Verification items for the finished model (mm, model axes). A direction names the side the tool comes from. Coordinates: 2 decimals unless noted, no trailing zeros. Order: outer loops, then holes, each group sorted by start corner. A loop starts at its lowest first (then second) coordinate and runs counter-clockwise, first axis right, second up. Notation, with made-up numbers: M 32.25,51 L 79.25,51 A15 cw 79.25,59 Z; hole C 24,2.5 d5. An arc over 180 degrees is marked long. Use one line per item in the form item = value. Start each with the question number.
```python
from build123d import *

# Parameters (mm, degrees)
CROQUIS1_W              = 50.8
CROQUIS1_H              = 25.5016
SALIENTE_EXTRUIR1_DEPTH = 3.175
CROQUIS2_W              = 25.5016
CROQUIS2_H              = 46.3804
SALIENTE_EXTRUIR2_DEPTH = 18.3388
CORTAR_EXTRUIR2_DEPTH   = 13.26
SALIENTE_EXTRUIR3_DEPTH = 1.27
CROQUIS6_W              = 25.5016
CROQUIS6_H              = 46.3804
SALIENTE_EXTRUIR4_DEPTH = 2.54
CROQUIS7_W              = 25.5016
CROQUIS7_H              = 3.175
SALIENTE_EXTRUIR5_DEPTH = 50.8
CROQUIS8_W              = 72.9488
CROQUIS8_H              = 46.3804
SALIENTE_EXTRUIR6_DEPTH = 3.175


with BuildPart() as part:
    # Croquis1 → Saliente-Extruir1 (new body)
    with BuildSketch(Plane(origin=(0, 23.1902, 0), x_dir=(1, 0, 0), z_dir=(0, 1, 0))):
        with Locations((76.2, 0)):
            Rectangle(CROQUIS1_W, CROQUIS1_H)
    extrude(amount=-SALIENTE_EXTRUIR1_DEPTH)

    # Croquis2 → Saliente-Extruir2 (add)
    with BuildSketch(Plane(origin=(101.6, 0, 0), x_dir=(0, 0, -1), z_dir=(1, 0, 0))):
        Rectangle(CROQUIS2_W, CROQUIS2_H)
    extrude(amount=SALIENTE_EXTRUIR2_DEPTH)

    # Croquis4 → Cortar-Extruir2 (cut)
    with BuildSketch(Plane(origin=(0, 7.26, 0), x_dir=(1, 0, 0), z_dir=(0, 1, 0))):
        Polygon((104.14, -5.08), (104.14, -12.7508), (116.94, -12.7508), (116.94, -9.1694), (119.9388, -6.6294), (119.9388, 6.6294), (116.94, 9.1694), (116.94, 12.7508), (104.14, 12.7508), (104.14, 5.08), (101.6, 2.54), (101.6, -2.54), align=None)
    extrude(amount=-CORTAR_EXTRUIR2_DEPTH, mode=Mode.SUBTRACT)

    # Croquis5 → Saliente-Extruir3 (add)
    with BuildSketch(Plane(origin=(119.9388, 0, 0), x_dir=(0, 0, -1), z_dir=(1, 0, 0))):
        Polygon((-12.7508, -23.1902), (-12.7508, -19.9644), (12.7, -19.9644), (12.7, 19.9644), (-12.7508, 19.9644), (-12.7508, 23.1902), (12.7508, 23.1902), (12.7508, -23.1902), align=None)
    extrude(amount=SALIENTE_EXTRUIR3_DEPTH)

    # Croquis6 → Saliente-Extruir4 (add)
    with BuildSketch(Plane(origin=(121.2088, 0, 0), x_dir=(0, 0, -1), z_dir=(1, 0, 0))):
        Rectangle(CROQUIS6_W, CROQUIS6_H)
        Polygon((6.651353306, 1.27), (6.651353306, 13.8938), (-6.607446694, 13.8938), (-6.607446694, -13.8938), (6.651353306, -13.8938), align=None, mode=Mode.SUBTRACT)
    extrude(amount=SALIENTE_EXTRUIR4_DEPTH)

    # Croquis7 → Saliente-Extruir5 (add)
    with BuildSketch(Plane.ZY.offset(-101.6)):
        with Locations((0, -21.6027)):
            Rectangle(CROQUIS7_W, CROQUIS7_H)
    extrude(amount=SALIENTE_EXTRUIR5_DEPTH)

    # Croquis8 → Saliente-Extruir6 (add)
    with BuildSketch(Plane(origin=(0, 0, -12.7508), x_dir=(-1, 0, 0), z_dir=(0, 0, -1))):
        with Locations((-87.2744, 0)):
            Rectangle(CROQUIS8_W, CROQUIS8_H)
    extrude(amount=SALIENTE_EXTRUIR6_DEPTH)


solid = part.part
```
1. Cross-section at D-D on x = 62. Enter the section's corners in (y, z), and give its area (3 significant figures).
2. Cross-section at B-B on z = -0.5. Enter the section's corners in (x, y).
3. Cross-section at A-A on y = 2.5. Enter the section's corners in (x, z).
4. Material ranges on line 1 along X through (y, z) = (3, -12); line 2 along Y through (x, z) = (67.5, 6.5); line 3 along X through (y, z) = (19.5, 10.5), recorded low to high.
5. Cross-section at C-C on z = -10. Enter the section's corners in (x, y).
6. Release check for a two-part mould opening along Z. For faces 1 (the flat face through (122, 13.894, 0)), 2 (the flat face through (77, -20.015, 0)), 3 (the flat face through (103.7, -0.1, 12.751)) record: pulls with the +Z half, pulls with the -Z half, needs draft (parallel to the pull), parting line crosses it, or undercut.
7. Tool access check on faces 4 (the flat face through (76, 20.015, 0)), 5 (the flat face through (122, 0, 6.607)), 6 (the flat face through (88, -23.19, -1)), 7 (the flat face through (104.14, 1, 9)), 8 (the flat face through (118.418, 0.723, 7.917)). Record the directions out of +Z, -Z, +X, -X, +Y, -Y that give a thin tool (end or side, any length) a straight path to the whole face; none if there is none.
8. Depth check by flat-ended pin: P1, Ø20, axis at x = 65.5, y = 7, coming from the +Z side; P2, Ø10, axis at x = 108.5, y = 0.5, coming from the +Z side; P3, Ø4, axis at y = -5.5, z = 0.5, coming from the +X side; P4, Ø1.8, axis at y = -1, z = 11, coming from the -X side. Enter the tip coordinate at first touch or a pass-through.
Final values:
q1.outline = M -23.19,-15.93 L 23.19,-15.93 L 23.19,12.75 L 20.02,12.75 L 20.02,-12.75 L -20.02,-12.75 L -20.02,12.75 L -23.19,12.75 Z
q1.area = 309 mm2
q2.outline = M 50.8,-23.19 L 123.75,-23.19 L 123.75,-13.89 L 121.21,-13.89 L 121.21,-19.96 L 119.94,-19.96 L 119.94,-6 L 101.6,-6 L 101.6,-20.02 L 50.8,-20.02 Z; M 50.8,20.02 L 101.6,20.02 L 101.6,7.26 L 119.94,7.26 L 119.94,19.96 L 121.21,19.96 L 121.21,13.89 L 123.75,13.89 L 123.75,23.19 L 50.8,23.19 Z
q3.outline = M 50.8,-15.93 L 123.75,-15.93 L 123.75,-6.65 L 121.21,-6.65 L 121.21,-12.7 L 119.94,-12.7 L 119.94,-6.63 L 116.94,-9.17 L 116.94,-12.75 L 104.14,-12.75 L 104.14,-5.08 L 101.6,-2.54 L 101.6,-12.75 L 50.8,-12.75 Z; M 101.6,2.54 L 104.14,5.08 L 104.14,12.75 L 101.6,12.75 Z; M 116.94,9.17 L 119.94,6.63 L 119.94,12.75 L 116.94,12.75 Z; M 121.21,6.61 L 123.75,6.61 L 123.75,12.75 L 121.21,12.75 Z
q4.line_1 = 101.6 to 104.14, 116.94 to 119.94, 121.21 to 123.75
q4.line_2 = -23.19 to -20.02, 20.02 to 23.19
q4.line_3 = 101.6 to 119.94, 121.21 to 123.75
q5.outline = M 50.8,-23.19 L 123.75,-23.19 L 123.75,23.19 L 50.8,23.19 L 50.8,20.02 L 101.6,20.02 L 101.6,-20.02 L 50.8,-20.02 Z; hole M 104.14,-6 L 116.94,-6 L 116.94,7.26 L 104.14,7.26 Z; hole M 119.94,-19.96 L 121.21,-19.96 L 121.21,19.96 L 119.94,19.96 Z
q6.face_1 = undercut
q6.face_2 = needs draft
q6.face_3 = pulls with the +Z half
q7.face_4 = +Z, -X
q7.face_5 = +X
q7.face_6 = +Z, -Z, +X, -X, -Y
q7.face_7 = +Z
q7.face_8 = none
q8.P1 = -12.75
q8.P2 = 12.75
q8.P3 = 119.94
q8.P4 = 101.6
